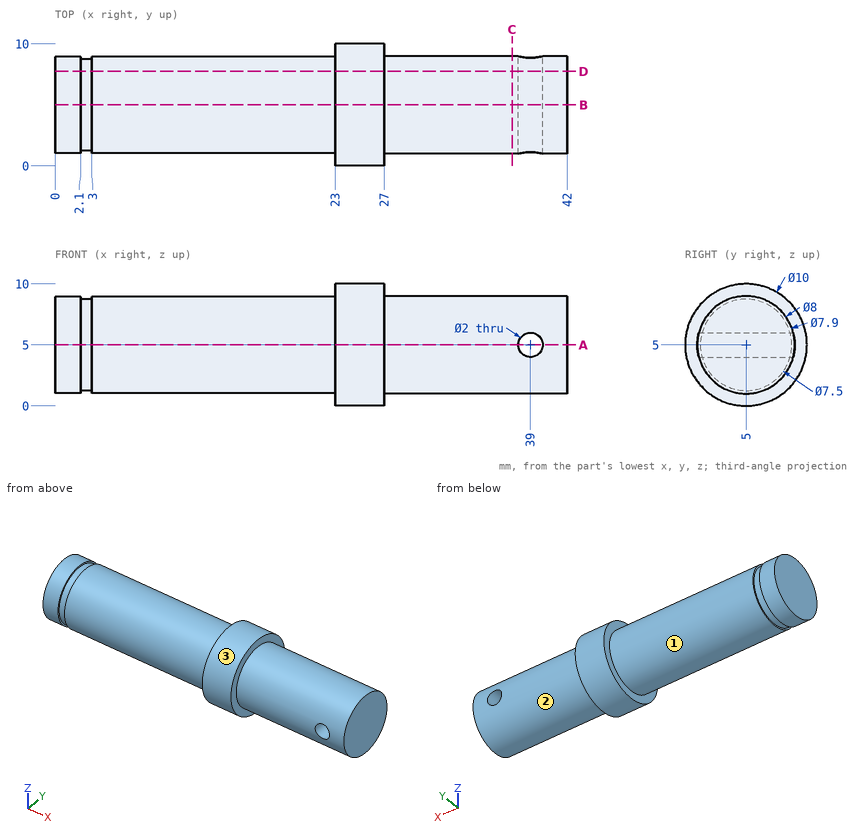
Here's the drawing with two shaded views (mm, measured from the low corner). I have some questions. A direction names the side the tool comes from. Coordinates: 2 decimals unless noted, no trailing zeros. Order: outer loops, then holes, each group sorted by start corner. A loop starts at its lowest first (then second) coordinate and runs counter-clockwise, first axis right, second up.
Q1. Please list where these lines run through material, in increasing order: L1, parallel to X at y = 4.5, z = 5; L2, parallel to Z at x = 39, y = 4.75; L3, parallel to Z at x = 39, y = 2.75.
Q2. Suppose I cut it at B-B on y = 5. Please give me the cut outline in (x, z), and give its area (3 significant figures).
Q3. Will these pins go through, and if not, where does the flat tip stop? pin 1 (1 mm diameter, centred on x = 35.5, z = 2.5, fed in from -Y); pin 2 (2.5 mm diameter, centred on x = 39, z = 5, fed in from -Y); pin 3 (2 mm diameter, centred on x = 33.5, y = 3.5, fed in from +Z).
Q4. Suppose I cut it at C-C on x = 37.5. Please give me the cut outline in (y, z), and give its area (3 significant figures).
Q5. Which directions (+Z, -Z, +X, -X, +Y, -Y) give clear straight access to the entire face, cutting with the end or side of a thin tool? Please do the marked faces 1, 2 and 3.
Q6. Suppose I cut it at D-D on y = 7.75. Please give me the cut outline in (x, z), and give its area (3 significant figures).
Q7. Suppose I cut it at A-A on z = 5. Please give me the cut outline in (x, y), and give its area (3 significant figures).
Answer:
1. L1: x = 0 to 38, 40 to 42
1. L2: z = 1.01 to 4, 6 to 8.99
1. L3: z = 1.69 to 4, 6 to 8.31
2. outline: (0, 1.05) - (2.1, 1.05) - (2.1, 1.25) - (3, 1.25) - (3, 1.05) - (23, 1.05) - (23, 0) - (27, 0) - (27, 1) - (42, 1) - (42, 9) - (27, 9) - (27, 10) - (23, 10) - (23, 8.95) - (3, 8.95) - (3, 8.75) - (2.1, 8.75) - (2.1, 8.95) - (0, 8.95) - close; hole circle Ø2 at (39, 5)
2. area: 338 mm2
3. pin 1: stops at y = 1.54
3. pin 2: stops at y = 1
3. pin 3: stops at z = 8.97
4. outline: circle Ø8 at (5, 5)
4. area: 50.3 mm2
5. face 1: -X
5. face 2: +X
5. face 3: +X, -X
6. outline: (0, 2.16) - (2.1, 2.16) - (2.1, 2.45) - (3, 2.45) - (3, 2.16) - (23, 2.16) - (23, 0.82) - (27, 0.82) - (27, 2.1) - (42, 2.1) - (42, 7.9) - (27, 7.9) - (27, 9.18) - (23, 9.18) - (23, 7.84) - (3, 7.84) - (3, 7.55) - (2.1, 7.55) - (2.1, 7.84) - (0, 7.84) - close; hole circle Ø2 at (39, 5)
6. area: 247 mm2
7. outline: (0, 1.05) - (2.1, 1.05) - (2.1, 1.25) - (3, 1.25) - (3, 1.05) - (23, 1.05) - (23, 0) - (27, 0) - (27, 1) - (38, 1) - (38, 9) - (27, 9) - (27, 10) - (23, 10) - (23, 8.95) - (3, 8.95) - (3, 8.75) - (2.1, 8.75) - (2.1, 8.95) - (0, 8.95) - close; (40, 1) - (42, 1) - (42, 9) - (40, 9) - close
7. area: 325 mm2
